Verification items for the finished model (mm, model axes). Face numbers are marked on the shaded views. A direction names the side the tool comes from. Round coordinates to 2 decimals unless told otherwise and drop trailing zeros. Order: outer loops, then holes, each group sorted by start corner. A loop starts at its lowest first (then second) coordinate and runs counter-clockwise, first axis right, second up. Notation, with made-up numbers: M 69,8.25 L 96,8.25 A32 cw 96,38.25 Z; hole C 51.5,24 d5. An arc over 180 degrees is marked long. Return JSON: item names as keys, results as strings. Group by question number.
from build123d import *

# Parameters (mm, degrees)
SKETCH1_W           = 27.94
SKETCH1_H           = 19.05
BOSS_EXTRUDE1_DEPTH = 138.4173
SKETCH5_R           = 3.556
BOSS_EXTRUDE2_DEPTH = 4.7752
SKETCH6_R           = 10.6045
SKETCH6_R_2         = 8.0645
BOSS_EXTRUDE3_DEPTH = 12.7
SKETCH8_R           = 8.0645
CUT_EXTRUDE2_DEPTH  = 151.882604283
SKETCH9_W           = 32.717360996
SKETCH9_H           = 24.765
CUT_EXTRUDE3_DEPTH  = 151.882604283
SKETCH10_R          = 1.27
BOSS_EXTRUDE4_DEPTH = 6.35
FILLET1_R           = 0.762


with BuildPart() as part:
    # Sketch1 → Boss-Extrude1 (new body)
    with BuildSketch(Plane(origin=(0, 0, 0), x_dir=(0, 0, -1), z_dir=(1, 0, 0))):
        Rectangle(SKETCH1_W, SKETCH1_H)
    extrude(amount=BOSS_EXTRUDE1_DEPTH)

    # Cut-Sweep1: sweep along a path in Sketch3
    with BuildLine(Plane.XY) as cut_sweep1_path:
        Line((138.4173, 9.525), (7.9502, 12.941401248))
    # Sketch2 → Cut-Sweep1 (sweep, cut)
    with BuildSketch(Plane(origin=(138.4173, 0, 0), x_dir=(0, 0, -1), z_dir=(1, 0, 0))):
        with BuildLine():
            Line((-9.525, 3.175), (-9.525, 9.525))
            Line((-9.525, 9.525), (9.525, 9.525))
            Line((9.525, 9.525), (9.525, 3.175))
            ThreePointArc((9.525, 3.175), (0, -6.35), (-9.525, 3.175))
        make_face()
    sweep(path=cut_sweep1_path.line, mode=Mode.SUBTRACT)

    # Sketch5 → Boss-Extrude2 (add)
    with BuildSketch(Plane(origin=(0, 0, -13.97), x_dir=(-1, 0, 0), z_dir=(0, 0, -1))):
        with BuildLine():
            Line((0, -9.525), (0, 9.525))
            Line((0, 9.525), (9.525, 9.525))
            ThreePointArc((9.525, 9.525), (19.05, 0), (9.525, -9.525))
            Line((9.525, -9.525), (0, -9.525))
        make_face()
        with Locations((9.525, 0)):
            Circle(SKETCH5_R, mode=Mode.SUBTRACT)
    extrude(amount=-BOSS_EXTRUDE2_DEPTH)

    # Sketch6 → Boss-Extrude3 (add)
    with BuildSketch(Plane.XZ.offset(9.525)):
        with Locations(Location((138.4173, 0, 0), (0, 0, 270))):
            Circle(SKETCH6_R)
        with Locations(Location((138.4173, 0, 0), (0, 0, 270))):
            Circle(SKETCH6_R_2, mode=Mode.SUBTRACT)
    extrude(amount=BOSS_EXTRUDE3_DEPTH)

    # Sketch8 → Cut-Extrude2 (cut, through all)
    with BuildSketch(Plane.XZ.offset(9.525)):
        with Locations(Location((138.4173, 0, 0), (0, 0, 270))):
            Circle(SKETCH8_R)
    extrude(amount=-CUT_EXTRUDE2_DEPTH, mode=Mode.SUBTRACT)

    # Sketch9 → Cut-Extrude3 (cut, through all)
    with BuildSketch(Plane.XZ.offset(9.525)):
        with Locations((154.775980498, 1.5875)):
            Rectangle(SKETCH9_W, SKETCH9_H)
    extrude(amount=CUT_EXTRUDE3_DEPTH, mode=Mode.SUBTRACT)

    # Sketch10 → Boss-Extrude4 (add)
    with BuildSketch(Plane(origin=(138.4173, 0, 0), x_dir=(0, 0, -1), z_dir=(1, 0, 0))):
        with Locations(Location((-11.43, -6.985, 0), (0, 0, 180))):
            Circle(SKETCH10_R)
        with Locations(Location((11.43, -6.985, 0), (0, 0, 180))):
            Circle(SKETCH10_R)
    extrude(amount=BOSS_EXTRUDE4_DEPTH)

    # Fillet1
    fillet1_edges = [part.edges().sort_by_distance(p)[0] for p in [
        (144.7673, -6.985, 10.16),
        (144.7673, -6.985, -12.7),
    ]]
    fillet(fillet1_edges, radius=FILLET1_R)


solid = part.part
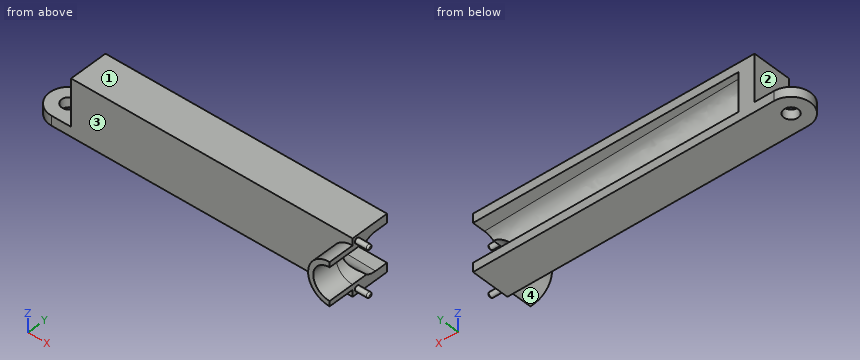
1. Cross-section at A-A (y = -13). Enter the section's corners in (x, z), plus the area to 3 significant figures.
2. Thickness scan on line 1 along Y through (x, z) = (25.5, 7.25) (3 decimals); line 2 along X through (y, z) = (0, -5.75); line 3 along Z through (x, y) = (-8, 6.5). Record the ranges inside material, lowest first. Write a range as from..to.
3. Go/stop test with flat-tipped pins: pin 1 (6 mm diameter, centred on y = -6, z = -7.5, fed in from +X); pin 2 (6 mm diameter, centred on y = 4, z = -0.5, fed in from +X); pin 3 (6 mm diameter, centred on y = -18, z = 1.5, fed in from -X). Record where each tip stops, or that it passes through.
4. Draft check along X on the marked faces 3 and 4. Enter one of: +X half, -X half, draft (parallel to the pull), parting line (faces both ways), or undercut.
5. Access from +Z, -Z, +X, -X, +Y, -Y to the whole of each face (thin tool, end or side, straight path). Record for the marked faces 1 and 2.
Computed:
{
 "1": {"outline": "M 138.42,-10.6 L 138.42,-8.06 A8.06 cw 138.42,8.06 L 138.42,10.6 A10.6 ccw Z", "area": "74.5 mm²"},
 "2": {"line 1": "y = -9.525..-0.046", "line 2": "x = 0..7.95", "line 3": "z = -13.97..-9.19"},
 "3": {"pin 1": "stops at x = 144.54", "pin 2": "stops at x = 7.95", "pin 3": "stops at x = 127.81"},
 "4": {"face 3": "draft", "face 4": "-X half"},
 "5": {"face 1": "+Z, +X, -X, +Y, -Y", "face 2": "+Z, -X, +Y, -Y"}
}
